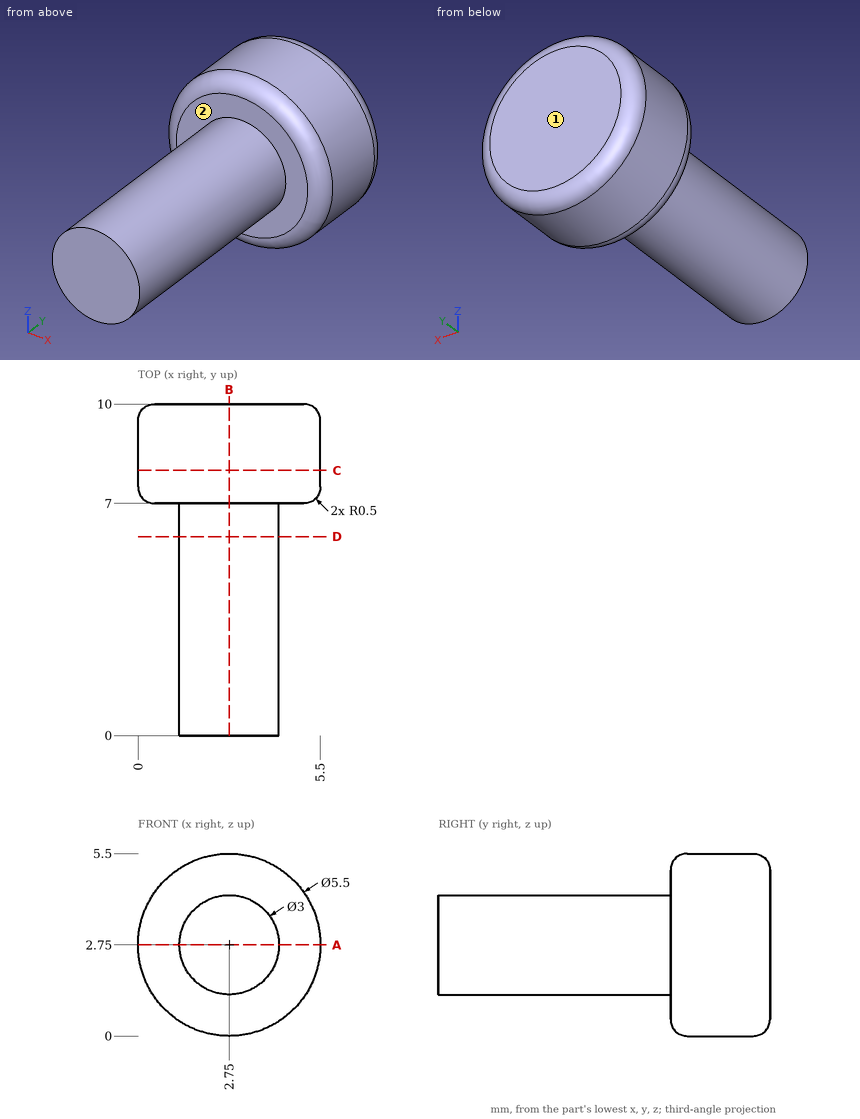
Here's the drawing with two shaded views (mm, measured from the low corner). I have some questions. A direction names the side the tool comes from. Give positions to 0.01 mm unless a question says otherwise; leave off trailing zeros. Write each loop counter-clockwise with the first axis right and the second up, starting at its lowest first coordinate (ties: lowest second). Pieces come first, ordered by that corner, then holes. Notation, with made-up numbers: (40.5, 18.25) -> (49.5, 18.25) arc R36 cw to (49.5, 57.25) -> close; hole circle Ø9 at (55, 58.5). An arc over 180 degrees is marked (long way). Use one line per item in the form item = value. Start each with the question number.
1. Imagine slicing it at D-D on y = 6. List the corners of the cut face in (x, z) for me, plus the area to 3 significant figures.
2. Imagine slicing it at A-A on z = 2.75. List the corners of the cut face in (x, y) for me, plus the area to 3 significant figures.
3. If I drill on L1, parallel to Y at x = 3, z = 0.75; L2, parallel to Z at x = 1.5, y = 3.5; L3, parallel to Z at x = 2.2, y = 1.5, over which ranges is the centre line in solid material (lowest first)?
4. On a 3-axis mill with a long thin cutter (end or side, diameter ignored), from which of +Z, -Z, +X, -X, +Y, -Y can I reach the whole of each face in a straight line? I mean the marked faces 1 and 2. Say none if no direction works.
5. Will these pins go through, and if not, where does the flat tip stop? pin 1 Ø1 at (x, y) = (3.5, 2) entering from -Z; pin 2 Ø3 at (y, z) = (8, 4.5) entering from -X; pin 3 Ø1 at (y, z) = (2, 3) entering from -X.
6. Imagine slicing it at B-B on x = 2.75. List the corners of the cut face in (y, z) for me, plus the area to 3 significant figures.
7. Imagine slicing it at C-C on y = 8. List the corners of the cut face in (x, z) for me, plus the area to 3 significant figures.
Entries:
q1.outline = circle Ø3 at (2.75, 2.75)
q1.area = 7.07 mm²
q2.outline = (0, 7.5) arc R0.5 ccw to (0.5, 7) -> (1.25, 7) -> (1.25, 0) -> (4.25, 0) -> (4.25, 7) -> (5, 7) arc R0.5 ccw to (5.5, 7.5) -> (5.5, 9.5) arc R0.5 ccw to (5, 10) -> (0.5, 10) arc R0.5 ccw to (0, 9.5) -> close
q2.area = 37.3 mm²
q3.L1 = 7 to 10
q3.L2 = 1.92 to 3.58
q3.L3 = 1.35 to 4.15
q4.face_1 = +Z, -Z, +X, -X, +Y
q4.face_2 = -Y
q5.pin_1 = 1.27
q5.pin_2 = 0.01
q5.pin_3 = 1.25
q6.outline = (0, 1.25) -> (7, 1.25) -> (7, 0.5) arc R0.5 ccw to (7.5, 0) -> (9.5, 0) arc R0.5 ccw to (10, 0.5) -> (10, 5) arc R0.5 ccw to (9.5, 5.5) -> (7.5, 5.5) arc R0.5 ccw to (7, 5) -> (7, 4.25) -> (0, 4.25) -> close
q6.area = 37.3 mm²
q7.outline = circle Ø5.5 at (2.75, 2.75)
q7.area = 23.8 mm²
